Print and shaded views of the part. All mm, measured from the part's lowest x, y and z. A direction names the side the tool comes from. Round coordinates to 2 decimals unless told otherwise and drop trailing zeros. Write each loop counter-clockwise with the first axis right and the second up, starting at its lowest first coordinate (ties: lowest second). Pieces come first, ordered by that corner, then holes.
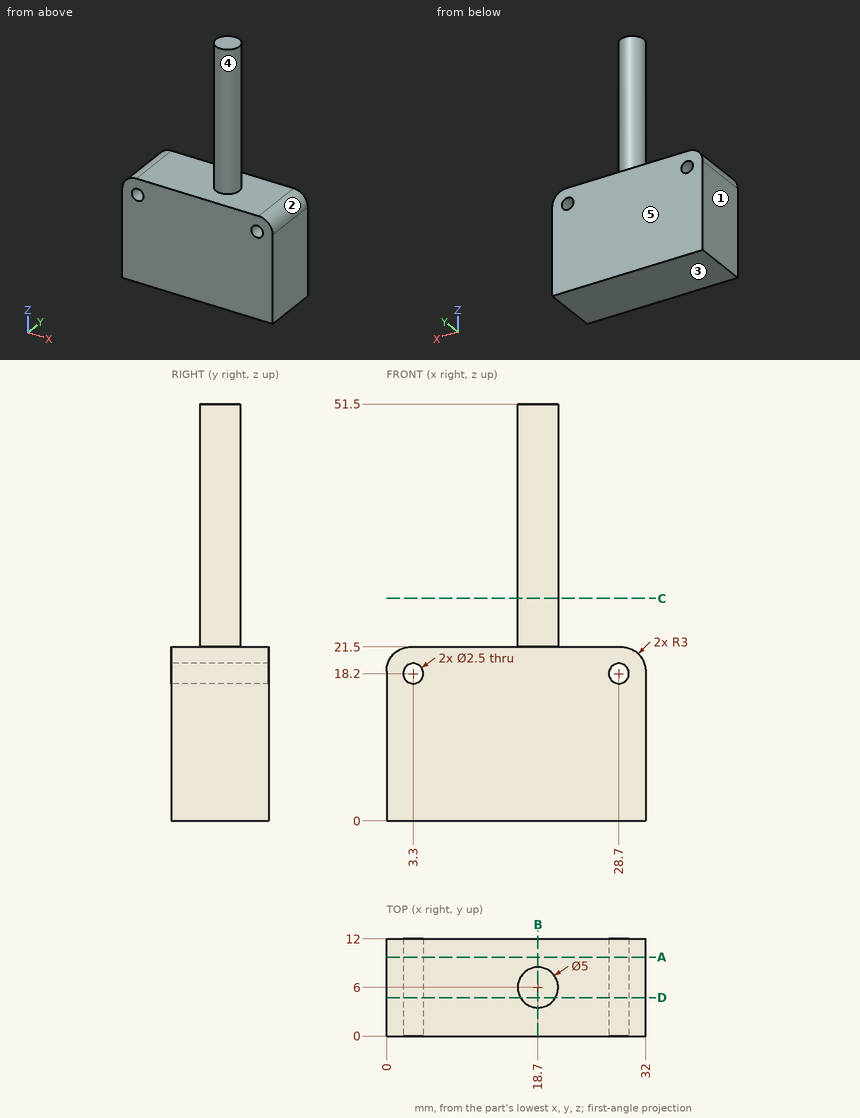
1) Slice it at B-B (x = 18.7). Write the cut outline in (y, z).
Results:
outline: (0, 0) - (12, 0) - (12, 21.5) - (8.5, 21.5) - (8.5, 51.5) - (3.5, 51.5) - (3.5, 21.5) - (0, 21.5) - close
2) Which spindle directions (+Z, -Z, +X, -X, +Y, -Y) get a long thin tool onto all of the face, cutting with end or side? Do the marked faces 4 and 5. Say none if no direction does.
Results:
face 4: +Z
face 5: +Z, -Z, +X, -X, +Y
3) Slice it at C-C (z = 27.5). Write the cut outline in (x, y).
Results:
outline: circle Ø5 at (18.7, 6)
4) Mould opens along Z. For the marked faces 1, 2 and 3 say: released by +Z, released by -Z, zero draft, split by the parting line, or undercut.
Results:
face 1: zero draft
face 2: released by +Z
face 3: released by -Z
5) Slice it at A-A (y = 9.75). Write the cut outline in (x, z), plus the area to 3 significant figures.
Results:
outline: (0, 0) - (32, 0) - (32, 18.5) arc R3 ccw to (29, 21.5) - (3, 21.5) arc R3 ccw to (0, 18.5) - close; hole circle Ø2.5 at (3.3, 18.2); hole circle Ø2.5 at (28.7, 18.2)
area: 674 mm2
6) Slice it at D-D (y = 4.75). Write the cut outline in (x, z), plus the area to 3 significant figures.
Results:
outline: (0, 0) - (32, 0) - (32, 18.5) arc R3 ccw to (29, 21.5) - (20.87, 21.5) - (20.87, 51.5) - (16.53, 51.5) - (16.53, 21.5) - (3, 21.5) arc R3 ccw to (0, 18.5) - close; hole circle Ø2.5 at (3.3, 18.2); hole circle Ø2.5 at (28.7, 18.2)
area: 804 mm2
7) Pin check, flat tips, straight feed: pin 1 Ø12 at (x, z) = (12, 45.5) entering from +Y; pin 2 Ø1 at (x, y) = (6, 7.5) entering from +Z. Stop position of each tip, or through.
Results:
pin 1: stops at y = 8.4
pin 2: stops at z = 21.5
8) Wall check: L1, parallel to X at y = 4.25, z = 18.2; L2, parallel to Z at x = 28.7, y = 7; L3, parallel to X at y = 4.5, z = 19. Give the ranges that are in metal, low to high.
Results:
L1: x = 0 to 2.05, 4.55 to 27.45, 29.95 to 32
L2: z = 0 to 16.95, 19.45 to 21.5
L3: x = 0.04 to 2.34, 4.26 to 27.74, 29.66 to 31.96
